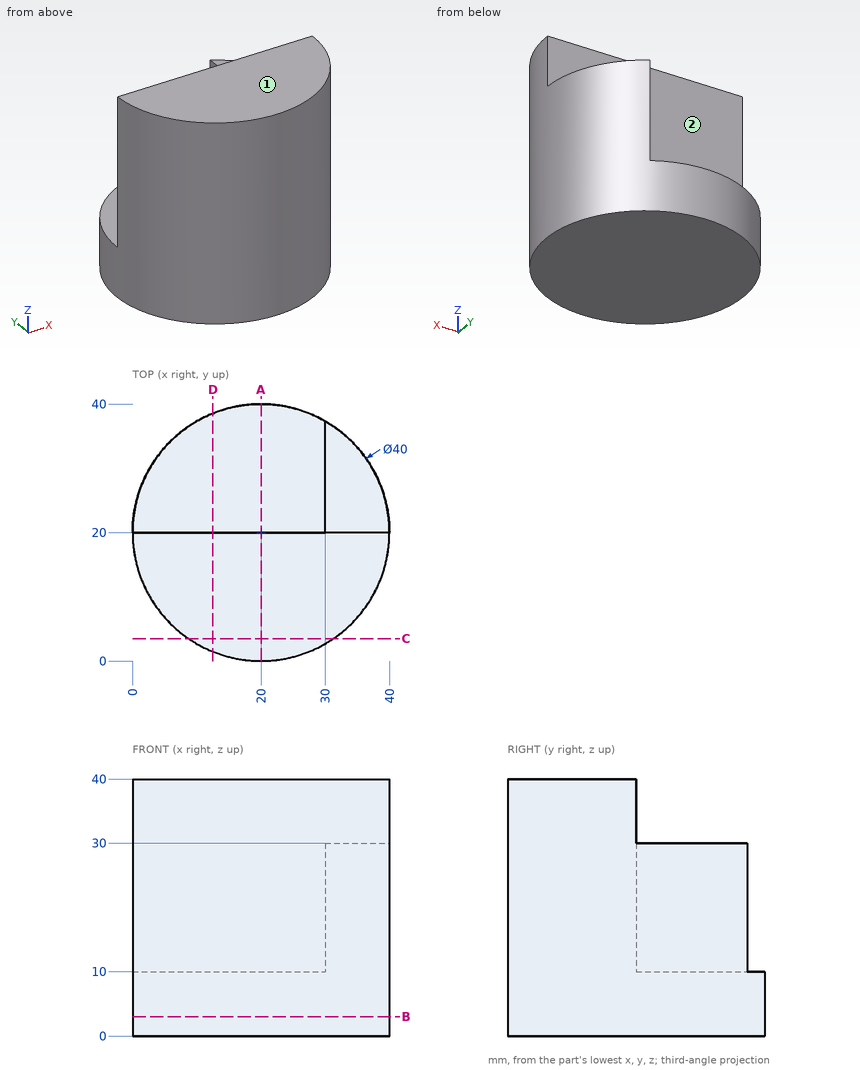
Geometry check sheet. Reference: drawing and pictorial views, mm from the part's lowest x, y, z. A direction names the side the tool comes from. Round coordinates to 2 decimals unless told otherwise and drop trailing zeros. Write each loop counter-clockwise with the first axis right and the second up, starting at its lowest first coordinate (ties: lowest second). Pieces come first, ordered by that corner, then holes.
1. Scan lines: L1, parallel to Z at x = 27, y = 36.5; L2, parallel to Z at x = 31.5, y = 21.5; L3, parallel to X at y = 20.5, z = 16. Record each from-to range of solid material in increasing order.
2. Section check D-D on x = 12.5. Enter the section's corners in (y, z), plus the area to 3 significant figures.
3. Section check A-A on x = 20. Enter the section's corners in (y, z).
4. Gauge pin test, flat ends, axial feed: P1, Ø1.5, axis at x = 25, z = 35.5, coming from the -Y side; P2, Ø3, axis at x = 29.5, z = 9.5, coming from the +Y side; P3, Ø24, axis at x = 26, z = 32, coming from the +Y side. Record the tip position at first contact, or that the pin passes through.
5. Section check C-C on y = 3.5. Enter the section's corners in (x, z), plus the area to 3 significant figures.
6. Access from +Z, -Z, +X, -X, +Y, -Y to the whole of each face (thin tool, end or side, straight path). Record for the marked faces 1 and 2.
7. Section check B-B on z = 3. Enter the section's corners in (x, y).
Answer:
1. L1: z = 0 to 10
1. L2: z = 0 to 30
1. L3: x = 30 to 39.99
2. outline: (1.46, 0) - (38.54, 0) - (38.54, 10) - (20, 10) - (20, 40) - (1.46, 40) - close
2. area: 927 mm2
3. outline: (0, 0) - (40, 0) - (40, 10) - (20, 10) - (20, 40) - (0, 40) - close
4. P1: stops at y = 0.46
4. P2: stops at y = 38.33
4. P3: stops at y = 37.32
5. outline: (8.7, 0) - (31.3, 0) - (31.3, 40) - (8.7, 40) - close
5. area: 904 mm2
6. face 1: +Z, +X, -X, +Y, -Y
6. face 2: +Z, -X, +Y
7. outline: circle Ø40 at (20, 20)
